Answer from the drawing. Dimensions are ordinates in mm from the lowest x, y and z of the part. A direction names the side the tool comes from. Round coordinates to 2 decimals unless told otherwise and drop trailing zeros. Write each loop counter-clockwise with the first axis right and the second up, starting at its lowest first coordinate (ties: lowest second). Pieces come first, ordered by that corner, then holes. Notation, with made-up numbers: (73.5, 34) - (111.5, 34) arc R20 cw to (111.5, 63) - close; hole circle Ø6 at (-35, -4.5). An arc over 180 degrees is marked (long way). Answer as CSV lines item,"result". Start each with the question number.
1) Find section D-D on z = 2.25. Determine the outline of the cut face in (x, y), then the cut area to 3 significant figures.
2) Each of these flat-tipped pins is pushed along its axis until it touches: pin 1 (2 mm diameter, centred on x = 6, y = 4.5, fed in from +Z); pin 2 (1.1 mm diameter, centred on y = 3.5, z = 0.5, fed in from +X). Where does it stop, or does it pass through?
3) Find section B-B on x = 2. Determine the outline of the cut face in (y, z), then the cut area to 3 significant figures.
4) For a pull along X with two mould halves and no side action, classify the marked faces 5, 6, 7 and 8 as +X half, -X half, draft (parallel to the pull), parting line (faces both ways), or undercut.
5) Consider line 1 along X through (y, z) = (0.5, 6); line 2 along Z through (x, y) = (2, 1.5); line 3 along X through (y, z) = (1.25, 5.5). Determine where each line is inside the solid, lowest interval first.
6) Find section A-A on z = 1.25. Determine the outline of the cut face in (x, y).
7) Which of the six approach directions +Z, -Z, +X, -X, +Y, -Y give full straight-line access (tool end or side, diameter ignored) to the marked faces 1, 2, 3 and 4?
8) Find section C-C on x = 3.69. Determine the outline of the cut face in (y, z).
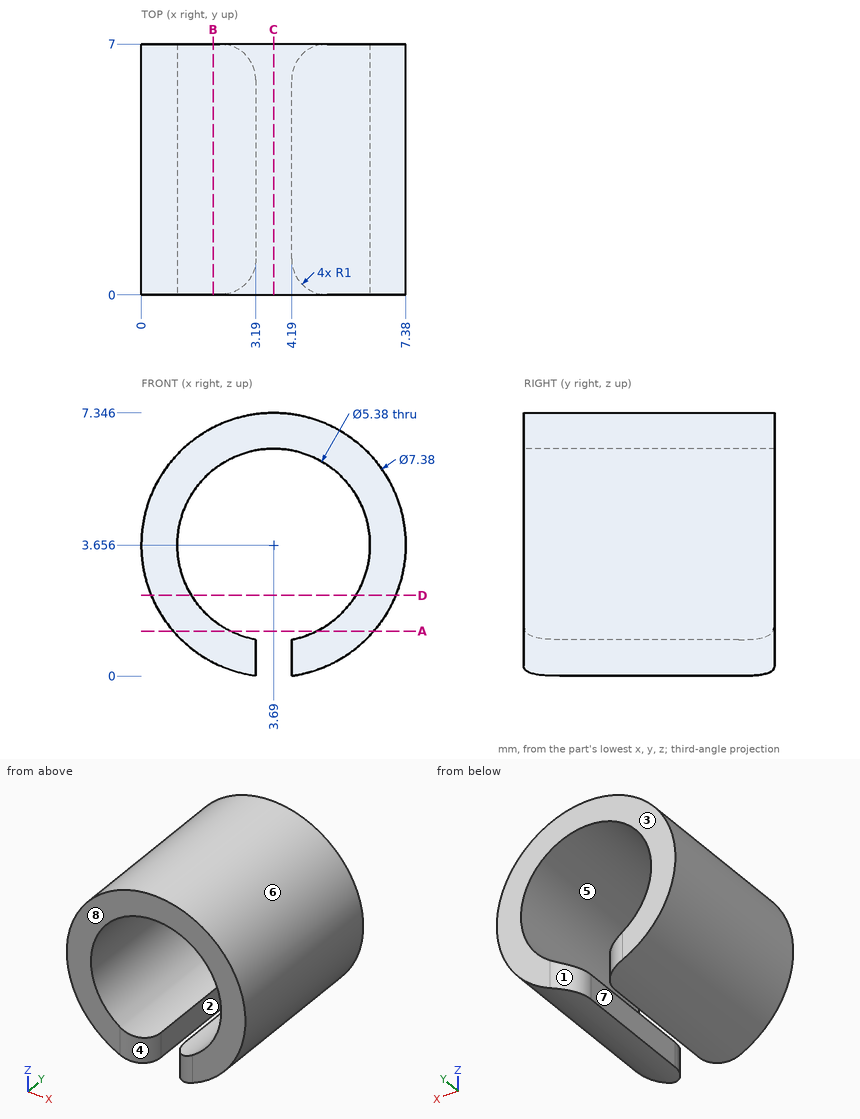
Check values:
1,outline,"(0.28, 0) - (1.4, 0) - (1.4, 7) - (0.28, 7) - close; (5.98, 0) - (7.1, 0) - (7.1, 7) - (5.98, 7) - close"
1,area,"15.7 mm^2"
2,pin 1,"stops at z = 7.11"
2,pin 2,"stops at x = 6.3"
3,outline,"(0, 0.38) - (7, 0.38) - (7, 1.56) - (0, 1.56) - close; (0, 5.75) - (7, 5.75) - (7, 6.94) - (0, 6.94) - close"
3,area,"16.6 mm^2"
4,face 5,"undercut"
4,face 6,"parting line"
4,face 7,"undercut"
4,face 8,"draft"
5,line 1,"x = 0.84 to 2.37, 5.01 to 6.54"
5,line 2,"z = 0.38 to 1.56, 5.75 to 6.94"
5,line 3,"x = 0.49 to 1.73, 5.65 to 6.89"
6,outline,"(0.89, 0) - (2.19, 0) arc R1 ccw to (2.49, 0.05) - (2.49, 6.95) arc R1 ccw to (2.19, 7) - (0.89, 7) - close; (4.89, 0.05) arc R1 ccw to (5.19, 0) - (6.49, 0) - (6.49, 7) - (5.19, 7) arc R1 ccw to (4.89, 6.95) - close"
7,face 1,"-Z, +Y"
7,face 2,"-Z, +Y, -Y"
7,face 3,"+Z, -Z, +X, -X, +Y"
7,face 4,"-Z, -Y"
8,outline,"(0, 6.35) - (7, 6.35) - (7, 7.35) - (0, 7.35) - close"
